Design review of the part built by this model. Coordinates are the model's own, in mm. Face numbers are marked on the shaded views. A direction names the side the tool comes from. Give positions to 0.01 mm unless a question says otherwise; leave off trailing zeros. Loops run counter-clockwise (first coordinate to the right, second up) from the corner with the lowest first, then second, coordinate; pieces in that order, holes last. Notation, with made-up numbers: (-6, 66.25) -> (50, 66.25) arc R14 ccw to (50, 82.25) -> close; hole circle Ø7 at (43, -3.5). An arc over 180 degrees is marked (long way). Use a Markdown table: item, result. Add a question column.
1. Add section B-B (y = -65). State the section outline as (x, z) points (3 decimals).
2. Add section D-D (x = 47.5). State the section outline as (y, z) points (3 decimals).
3. For the marked faces 1 and 2, list the 3-axis set-ups (+Z, -Z, +X, -X, +Y, -Y) from which the entire face can be reached by the end or side of a thin tool; tool diameter is ignored.
4. To check wall thickness, follow line 1 (Y direction, x = 0, z = 0.9); line 2 (Y direction, x = 138.5, z = -8.75); line 3 (Z direction, x = 1.5, y = -60.5) (3 decimals). State the ranges of each line that lie inside material, in increasing order.
5. Add section C-C (x = 120). State the section outline as (y, z) points (3 decimals), and give its area (3 significant figures).
6. For pin 1 Ø8 at (x, z) = (130.5, -13) entering from +Y; pin 2 Ø5 at (x, y) = (51, 46) entering from -Z; pin 3 Ø17 at (x, y) = (0, 84.94) entering from +Z; pin 4 Ø5 at (y, z) = (87, -1.5) entering from +X, all flat-tipped, find the tip position at first contact; note any pin that passes through.
7. Add section A-A (x = 0). State the section outline as (y, z) points (3 decimals), and give its area (3 significant figures).
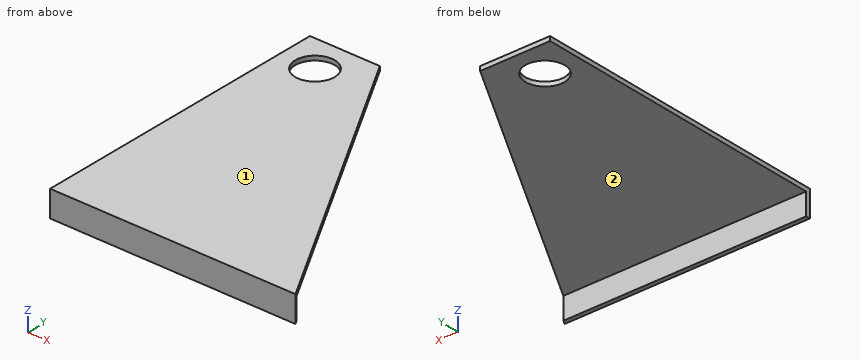
Autodesk Inventor part; units mm, degrees
ref_plane "YZ Plane" through (0, 0, 0) normal (1, 0, 0) x (0, 1, 0)
ref_plane "XZ Plane" through (0, 0, 0) normal (0, 1, 0) x (-1, 0, 0)
ref_plane "XY Plane" through (0, 0, 0) normal (0, 0, 1) x (1, 0, 0)
sketch "Sketch1" plane through (0, 0, 0) normal (0, 0, 1) x (1, 0, 0)
  line L0 (25.4, -110.3376) -> (-25.4, -110.3376)
  line L1 (-25.4, -110.3376) -> (-25.4, 110.3376)
  line L2 (-25.4, 110.3376) -> (25.4, 110.3376)
  line L3 (25.4, 110.3376) -> (25.4, -110.3376)
  line L4 (25.4, -110.3376) -> (-25.4, 110.3376) construction
  line L5 (-25.4, -110.3376) -> (25.4, 110.3376) construction
  line L6 (25.4, 110.3376) -> (152.8069, -110.3376)
  line L7 (25.4, 110.3376) -> (280.2138, 110.3376) construction
  line L8 (152.8069, -110.3376) -> (25.4, -110.3376)
  point P0 (0, 0)
  dimension "d0" = 50.8
  dimension "d1" = 220.6752
  dimension "d2" = 60
extrude "Extrusion1" add sketch "Sketch1" along normal blind 3.175
sketch "Sketch2" plane through (0, 0, 3.175) normal (0, 0, 1) x (1, 0, 0)
  line L0 (152.8069, -110.3376) -> (25.4, 110.3376)
  line L1 (-25.4, -110.3376) -> (152.8069, -110.3376)
  line L2 (152.8069, -107.1626) -> (-25.4, -107.1626)
  line L3 (-25.4, -107.1626) -> (-25.4, -110.3376)
  line L4 (150.9738, -107.1626) -> (152.8069, -110.3376)
  point P0 (0, 0)
  dimension "d5" = 3.175
extrude "Extrusion2" add sketch "Sketch2" against normal blind 19.05
sketch "Sketch3" plane through (0, 0, 3.175) normal (0, 0, 1) x (1, 0, 0)
  line L0 (-25.4, 110.3376) -> (0, 110.3376)
  line L1 (0, 110.3376) -> (0, 84.9376)
  line L2 (0, 84.9376) -> (-25.4, 84.9376)
  line L3 (-25.4, 84.9376) -> (-25.4, 110.3376)
  circle A0 centre (0, 84.9376) radius 14.2875
  point P0 (0, 0)
  dimension "d8" = 25.4
  dimension "d9" = 25.4
  dimension "d10" = 28.575
extrude "Extrusion3" cut sketch "Sketch3" against normal blind 25.4 contours A0 L2 L1 | L1 L2 A0
properties part number "RPlate"
Taken from the geometry:
| question | item | result |
|---|---|---|
| 1 | outline | (-25.4, 0) -> (126.631, 0) -> (126.631, 3.175) -> (-25.4, 3.175) -> close |
| 2 | outline | (-110.338, -15.875) -> (-107.163, -15.875) -> (-107.163, 0) -> (72.059, 0) -> (72.059, 3.175) -> (-110.338, 3.175) -> close |
| 3 | face 1 | +Z, +X, -X, +Y, -Y |
| 3 | face 2 | -Z, +X, -X, +Y |
| 4 | line 1 | y = -110.34 to 70.65, 99.23 to 110.34 |
| 4 | line 2 | y = -110.34 to -107.16 |
| 4 | line 3 | z = 0 to 3.175 |
| 5 | outline | (-110.338, -15.875) -> (-107.163, -15.875) -> (-107.163, 0) -> (-53.514, 0) -> (-53.514, 3.175) -> (-110.338, 3.175) -> close |
| 5 | area | 231 mm^2 |
| 6 | pin 1 | stops at y = -107.16 |
| 6 | pin 2 | stops at z = 0 |
| 6 | pin 3 | passes through |
| 6 | pin 4 | stops at x = 40.03 |
| 7 | outline | (-110.338, -15.875) -> (-107.163, -15.875) -> (-107.163, 0) -> (70.65, 0) -> (70.65, 3.175) -> (-110.338, 3.175) -> close; (99.225, 0) -> (110.338, 0) -> (110.338, 3.175) -> (99.225, 3.175) -> close |
| 7 | area | 660 mm^2 |
